from build123d import *

# Parameters (mm, degrees)
BOSS_EXTRUDE1_DEPTH = 17
SKETCH3_W           = 10
SKETCH3_H           = 23
BOSS_EXTRUDE2_DEPTH = 17
SKETCH4_R           = 1.8
CUT_EXTRUDE1_DEPTH  = 42.475618626
SKETCH5_W           = 22.6
SKETCH5_H           = 6
BOSS_EXTRUDE3_DEPTH = 25
SKETCH6_R           = 1.8
CUT_EXTRUDE2_DEPTH  = 53.324521174
SKETCH7_R           = 3.5
CUT_EXTRUDE3_DEPTH  = 2


with BuildPart() as part:
    # Sketch2 → Boss-Extrude1 (new body)
    with BuildSketch(Plane.XY):
        Polygon((-7.526296722, 9.460038951), (-7.526296722, -5.139961049), (7.073703278, -5.139961049), (7.073703278, 9.460038951), (1.960317302, 9.460038951), (1.960317302, 20.960038951), (5.460317302, 20.960038951), (5.460317302, 12.960038951), (11.073703278, 12.960038951), (11.073703278, -11.139961049), (-11.526296722, -11.139961049), (-11.526296722, 12.960038951), (-5.912910746, 12.960038951), (-5.912910746, 20.960038951), (-2.412910746, 20.960038951), (-2.412910746, 9.460038951), align=None)
    extrude(amount=BOSS_EXTRUDE1_DEPTH)

    # Sketch3 → Boss-Extrude2 (add)
    with BuildSketch(Plane.XY.offset(17)):
        with Locations((-0.226296722, -22.639961049)):
            Rectangle(SKETCH3_W, SKETCH3_H)
    extrude(amount=-BOSS_EXTRUDE2_DEPTH)

    # Sketch4 → Cut-Extrude1 (cut, through all)
    with BuildSketch(Plane(origin=(4.773703278, 0, 0), x_dir=(0, 0, -1), z_dir=(1, 0, 0))):
        with Locations(Location((-8.5, -28.139961049, 0), (0, 0, 90))):
            Circle(SKETCH4_R)
        with Locations(Location((-8.5, 17.360038951, 0), (0, 0, 90))):
            Circle(SKETCH4_R)
    extrude(amount=-CUT_EXTRUDE1_DEPTH, mode=Mode.SUBTRACT)

    # Sketch5 → Boss-Extrude3 (add)
    with BuildSketch(Plane.XY.offset(17)):
        with Locations((-0.226296722, -8.139961049)):
            Rectangle(SKETCH5_W, SKETCH5_H)
    extrude(amount=BOSS_EXTRUDE3_DEPTH)

    # Sketch6 → Cut-Extrude2 (cut, through all)
    with BuildSketch(Plane(origin=(0, -5.139961049, 0), x_dir=(1, 0, 0), z_dir=(0, 1, 0))):
        with Locations(Location((-0.226296722, -36, 0), (0, 0, 180))):
            Circle(SKETCH6_R)
        with Locations(Location((-0.226296722, -28, 0), (0, 0, 180))):
            Circle(SKETCH6_R)
        with Locations(Location((-0.226296722, -20, 0), (0, 0, 180))):
            Circle(SKETCH6_R)
    extrude(amount=-CUT_EXTRUDE2_DEPTH, mode=Mode.SUBTRACT)

    # Sketch7 → Cut-Extrude3 (cut)
    with BuildSketch(Plane(origin=(0, -5.139961049, 0), x_dir=(1, 0, 0), z_dir=(0, 1, 0))):
        with Locations(Location((-0.226296722, -36, 0), (0, 0, 180))):
            Circle(SKETCH7_R)
        with Locations(Location((-0.226296722, -28, 0), (0, 0, 180))):
            Circle(SKETCH7_R)
        with Locations(Location((-0.226296722, -20, 0), (0, 0, 180))):
            Circle(SKETCH7_R)
    extrude(amount=-CUT_EXTRUDE3_DEPTH, mode=Mode.SUBTRACT)


solid = part.part
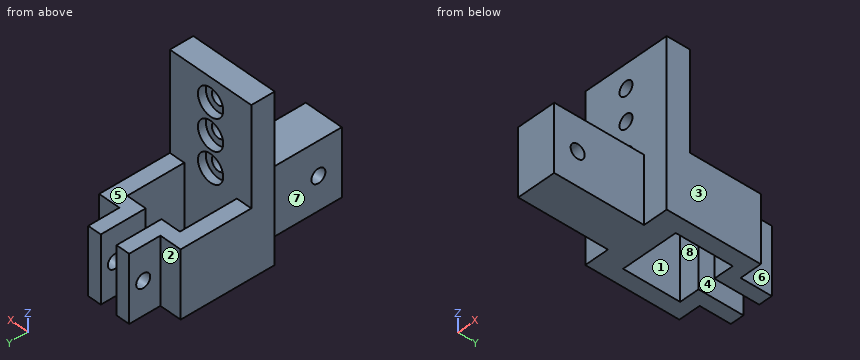
Can you work these out from the model? Positions are in its coordinate system, mm. Face numbers are marked on the shaded views. A direction names the side the tool comes from. Give positions to 0.01 mm unless a question says otherwise; leave off trailing zeros. Order: outer loops, then holes, each group sorted by start corner. A loop starts at its lowest first (then second) coordinate and runs counter-clockwise, first axis right, second up. Notation, with made-up numbers: M 30,60 L 47,60 A13 ccw 47,65 Z; hole C 63.5,-19 d5. An arc over 180 degrees is marked long. Use a Markdown table: item, result. Add a question column.
Item 1: Suppose I cut it at C-C (x = -0.25). Count the separate pieces of the cut face and the enclosed holes in it, then the cut area to 3 significant figures.
Item 2: Suppose I cut it at B-B (x = -6.75). List the corners of the cut face in (y, z) for me, then the cut area to 4 significant figures.
Item 3: For the marked faces 4, 5, 6, 7 and 8, which set-ups out of +Z, -Z, +X, -X, +Y, -Y let a thin tool reach every point of the face, with its end or its side?
Item 4: Suppose I cut it at A-A (z = 36). List the corners of the cut face in (x, y) for me, then the cut area to 3 significant figures.
Item 5: We'd pull the mould along Y, two halves only. Please class the marked faces 1, 2 and 3: +Y half, -Y half, draft (parallel to the pull), parting line (faces both ways), or undercut.
Item 6: Suppose I cut it at D-D (y = -28). List the corners of the cut face in (x, z) for me.
Item 7: If I drill on L1, parallel to X at y = 14, z = 15; L2, parallel to X at y = -4, z = 9.5; L3, parallel to Y at x = 6, z = 11.5, over which ranges is the centre line in solid material (lowest first)? Write a range as [from, to].
Item 8: Will these pins go through, and if not, where does the flat tip stop? pin 1 (3 mm diameter, centred on x = -4.5, y = 6.5, fed in from -Z); pin 2 (3.5 mm diameter, centred on x = -1.5, z = 35.5, fed in from +Y); pin 3 (1.5 mm diameter, centred on x = 8.5, z = 14, fed in from +Y); pin 4 (6 mm diameter, centred on x = 1.5, z = 30, fed in from +Y).
Answer sheet:
| question | item | result |
|---|---|---|
| 1 | separate pieces | 4 |
| 1 | enclosed holes | 1 |
| 1 | area | 548 mm² |
| 2 | outline | M -11.14,0 L -5.14,0 L -5.14,42 L -11.14,42 Z; M 9.46,0 L 12.96,0 L 12.96,17 L 9.46,17 Z |
| 2 | area | 311.5 mm² |
| 3 | face 4 | +Z, -Z, +Y |
| 3 | face 5 | +Z, +X, -X, +Y |
| 3 | face 6 | +Z, -Z, +X, +Y |
| 3 | face 7 | +Z, -Z, -X, -Y |
| 3 | face 8 | +Z, -Z |
| 4 | outline | M -11.53,-11.14 L -2.03,-11.14 L -2.03,-7.14 L -3.73,-7.14 L -3.73,-5.14 L -11.53,-5.14 Z; M 1.57,-11.14 L 11.07,-11.14 L 11.07,-5.14 L 3.27,-5.14 L 3.27,-7.14 L 1.57,-7.14 Z |
| 4 | area | 107 mm² |
| 5 | face 1 | undercut |
| 5 | face 2 | +Y half |
| 5 | face 3 | draft |
| 6 | outline | M -5.23,0 L 4.77,0 L 4.77,6.71 L -5.23,6.71 Z; M -5.23,10.29 L 4.77,10.29 L 4.77,17 L -5.23,17 Z |
| 7 | L1 | x = [-5.91, -2.41], [1.96, 5.46] |
| 7 | L2 | x = [-11.53, -7.53], [7.07, 11.07] |
| 7 | L3 | y = [-11.14, -5.14], [9.46, 12.96] |
| 8 | pin 1 | passes through |
| 8 | pin 2 | stops at y = -7.14 |
| 8 | pin 3 | stops at y = 12.96 |
| 8 | pin 4 | stops at y = -5.14 |
